Can you work these out from the model? Positions are in its coordinate system, mm. Face numbers are marked on the shaded views. A direction names the side the tool comes from. Give positions to 0.01 mm unless a question says otherwise; leave off trailing zeros. Loops run counter-clockwise (first coordinate to the right, second up) from the corner with the lowest first, then second, coordinate; pieces in that order, holes last. Notation, with made-up numbers: M -16.75,65.5 L -5.75,65.5 A16 ccw -5.75,96.5 Z; hole C 9.5,87 d1. An arc over 180 degrees is marked long. Answer as a JSON object with one key per item and string values.
Autodesk Fusion 360 part; units mm, degrees
sketch "Sketch1" plane through (0, 0, 0) normal (0, 0, 1) x (1, 0, 0)
  line L0 (15.55, 18.25) -> (-15.55, 18.25)
  line L1 (-15.55, 18.25) -> (-15.55, -18.25)
  line L2 (-15.55, -18.25) -> (15.55, -18.25)
  line L3 (15.55, -18.25) -> (15.55, 18.25)
  line L4 (15.55, 18.25) -> (-15.55, -18.25) construction
  line L5 (-15.55, 18.25) -> (15.55, -18.25) construction
  dimension "d1" = 31.1
  dimension "d2" = 36.5
extrude "Extrude1" add sketch "Sketch1" along normal blind 50
sketch "Sketch2" plane through (0, 0, 50) normal (0, 0, 1) x (-1, 0, 0)
  line L0 (-15.55, 18.25) -> (-15.55, -18.25)
  line L1 (-15.55, -18.25) -> (15.55, -18.25)
  line L2 (15.55, -18.25) -> (15.55, 18.25)
  line L3 (15.55, 18.25) -> (-15.55, 18.25)
  circle A0 centre (0, 0) radius 11
  dimension "d5" = 22
extrude "Extrude2" cut sketch "Sketch2" against normal blind 16 contours A0
extrude "Extrude3" cut 1 faces at (-2.9076, 1.5312, 34) along direction (0, 0, -1) blind 69.898
sketch "Sketch3" plane through (0, 0, 50) normal (0, 0, 1) x (-1, 0, 0)
  circle A0 centre (0, 0) radius 11
  line L0 (-15.55, 18.25) -> (-15.55, -18.25)
  line L1 (-15.55, -18.25) -> (15.55, -18.25)
  line L2 (15.55, -18.25) -> (15.55, 18.25)
  line L3 (15.55, 18.25) -> (-15.55, 18.25)
  line L4 (-17.55, -20.25) -> (17.55, -20.25)
  line L5 (17.55, -20.25) -> (17.55, 20.25)
  line L6 (17.55, 20.25) -> (-17.55, 20.25)
  line L7 (-17.55, 20.25) -> (-17.55, -20.25)
  dimension "d10" = 2
extrude "Extrude4" add sketch "Sketch3" against normal blind 4 contours L0 L1 L2 L3 | L4 L5 L6 L7
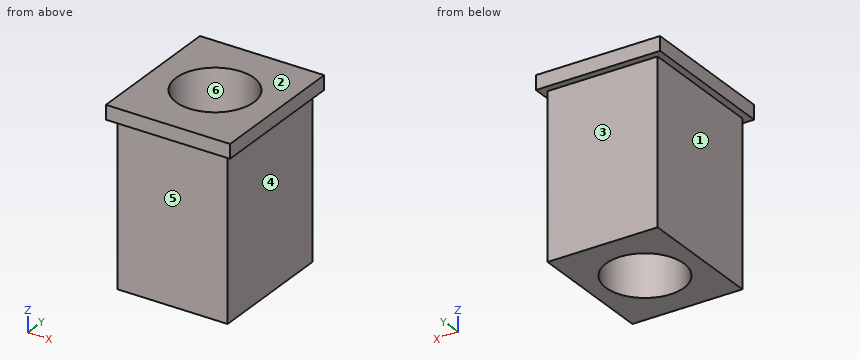
1) Will these pins go through, and if not, where does the flat tip stop? pin 1 Ø8 at (y, z) = (-9, 38) entering from -X; pin 2 Ø2 at (x, z) = (-12.5, 15) entering from +Y; pin 3 Ø15.5 at (x, z) = (4, 16) entering from -Y.
Answer list:
{"pin 1": "x = -15.55", "pin 2": "y = 18.25", "pin 3": "y = -18.25"}
2) Please list where these lines run through material, in increasing order: line 1 along X through (y, z) = (0, 36); line 2 along Y through (x, z) = (0, 28); line 3 along Y through (x, z) = (15, 4). Write a range as from..to.
Answer list:
{"line 1": "-15.55..-11, 11..15.55", "line 2": "-18.25..-11, 11..18.25", "line 3": "-18.25..18.25"}
3) Suppose I cut it at B-B, the plane x = 0. Write out the boundary of the cut face in (y, z).
Answer list:
{"outline": "M -20.25,46 L -18.25,46 L -18.25,0 L -11,0 L -11,50 L -20.25,50 Z; M 11,0 L 18.25,0 L 18.25,46 L 20.25,46 L 20.25,50 L 11,50 Z"}
4) Suppose I cut it at C-C, the plane y = 14. Write out the boundary of the cut face in (x, z), and give its area (3 significant figures).
Answer list:
{"outline": "M -17.55,46 L -15.55,46 L -15.55,0 L 15.55,0 L 15.55,46 L 17.55,46 L 17.55,50 L -17.55,50 Z", "area": "1,570 mm^2"}
5) For the marked faces 1, 2 and 3, which set-ups out of +Z, -Z, +X, -X, +Y, -Y let a thin tool reach every point of the face, with its end or its side?
Answer list:
{"face 1": "-Z, -X, +Y, -Y", "face 2": "+Z, +X, -X, +Y, -Y", "face 3": "-Z, +X, -X, +Y"}
6) If we mould it in two halves opening along Y, with no side actions, what happens to the marked faces 4, 5 and 6? For each: +Y half, -Y half, draft (parallel to the pull), parting line (faces both ways), or undercut.
Answer list:
{"face 4": "draft", "face 5": "-Y half", "face 6": "undercut"}
7) Suppose I cut it at D-D, the plane z = 12.5. Write out the boundary of the cut face in (x, y).
Answer list:
{"outline": "M -15.55,-18.25 L 15.55,-18.25 L 15.55,18.25 L -15.55,18.25 Z; hole C 0,0 d22"}
8) Suppose I cut it at A-A, the plane y = 0. Write out the boundary of the cut face in (x, z).
Answer list:
{"outline": "M -17.55,46 L -15.55,46 L -15.55,0 L -11,0 L -11,50 L -17.55,50 Z; M 11,0 L 15.55,0 L 15.55,46 L 17.55,46 L 17.55,50 L 11,50 Z"}
